The model under review builds one solid part; all positions refer to its coordinate system, in mm. Face numbers are marked on the shaded views. A direction names the side the tool comes from. Round coordinates to 2 decimals unless told otherwise and drop trailing zeros. Order: outer loops, then holes, each group sorted by start corner. A loop starts at its lowest first (then second) coordinate and runs counter-clockwise, first axis right, second up. Notation, with made-up numbers: M -16.75,-34 L -5.75,-34 A13 ccw -5.75,-19 Z; hole C 64,54 d11. An arc over 180 degrees is marked long. Answer as a JSON object with one key per item and string values. Group by question number.
1) For the marked faces 4, 5, 6 and 7, list the 3-axis set-ups (+Z, -Z, +X, -X, +Y, -Y) from which the entire face can be reached by the end or side of a thin tool; tool diameter is ignored.
2) The part is to be moulded in two halves that separate along X. For the marked faces 1, 2 and 3, say which applies: +X half, -X half, draft (parallel to the pull), parting line (faces both ways), or undercut.
3) Insertion check: pin 1 Ø0.5 at (y, z) = (6.5, 0) entering from -X (3 decimals); pin 2 Ø1.4 at (x, y) = (0, 6.5) entering from -Z; pin 3 Ø0.9 at (y, z) = (4, 0) entering from +X. Each pin has a flat end and moves straight along its axis. Give the tip position at first contact, or say it passes through.
4) Consider section A-A, the plane z = 0. Write out the cut boundary in (x, y) (1 decimal).
5) To check wall thickness, follow line 1 (Y direction, x = 0, z = 0) (3 decimals); line 2 (X direction, y = 4.25, z = -0.75); line 3 (Y direction, x = 0, z = -1.2). State the ranges of each line that lie inside material, in increasing order.
6) Consider section B-B, the plane x = 0. Write out the cut boundary in (y, z) (1 decimal), then the cut area to 3 significant figures.
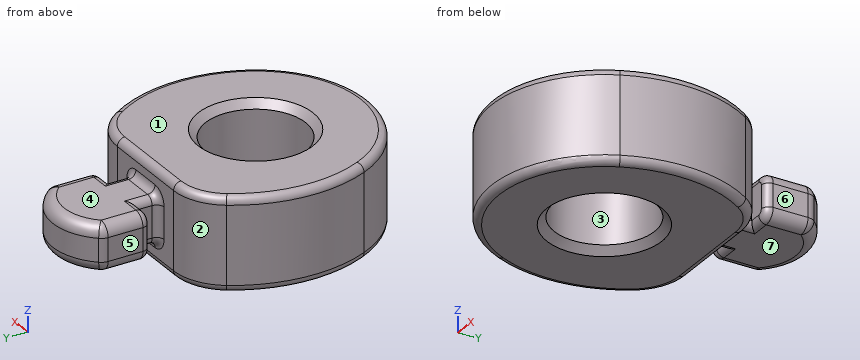
```python
from build123d import *

# Parameters (mm, degrees)
F1_DEPTH = 1.5875
F2_DEPTH = 3.175
F3_R     = 3.17499
F4_R     = 0.79375
F6_DEPTH = 3.175
F7_R     = 0.508
F8_R     = 0.508
F9_SIZE  = 0.508


# Not quite as in the source:
# - a fillet or chamfer is up to 0.001 mm smaller than in the source, because OpenCascade refuses the exact size
# - a feature names something its author has since deleted; it is built from what else it names


with BuildPart() as f1:
    # F0 (on Top) → F1 (new body, symmetric)
    with BuildSketch(Plane.XY):
        with BuildLine():
            Line((3.175, 4.7625), (3.175, 7.9375))
            ThreePointArc((3.175, 7.9375), (0, 9.525), (-3.175, 7.9375))
            Line((-3.175, 7.9375), (-3.175, 4.7625))
            Line((-3.175, 4.7625), (-1.5875, 4.7625))
            Line((-1.5875, 4.7625), (-1.5875, 3.175))
            Line((-1.5875, 3.175), (1.5875, 3.175))
            Line((1.5875, 3.175), (1.5875, 4.7625))
            Line((1.5875, 4.7625), (3.175, 4.7625))
        make_face()
    extrude(amount=F1_DEPTH, both=True)

    # F0 (on Top) → F2 (join, symmetric)
    with BuildSketch(Plane.XY):
        Polygon((6.35, 3.175), (1.5875, 3.175), (-1.5875, 3.175), (-6.35, 3.175), (-6.35, 0), (6.35, 0), align=None)
    extrude(amount=F2_DEPTH, both=True)

    # F3 (radius 3.175 in the source; OpenCascade refuses exactly that, so slightly less here)
    f3_edges = [f1.edges().sort_by_distance(p)[0] for p in [
        (6.35, 3.175, 0),
        (-6.35, 3.175, 0),
    ]]
    fillet(f3_edges, radius=F3_R)

    # F4
    f4_edges = [f1.edges().sort_by_distance(p)[0] for p in [
        (0, 9.525, -1.5875),
        (0, 9.525, 1.5875),
        (3.175, 6.35, -1.5875),
        (3.175, 6.35, 1.5875),
        (-3.175, 6.35, -1.5875),
        (-3.175, 6.35, 1.5875),
        (3.175, 7.9375, 0),
        (-3.175, 7.9375, 0),
    ]]
    fillet(f4_edges, radius=F4_R)

    # F5 (on Top) → F6 (join, symmetric)
    with BuildSketch(Plane.XY):
        with BuildLine():
            Line((1.5875, 3.175), (-1.5875, 3.175))
            ThreePointArc((-1.5875, 3.175), (-6.8727430801, -0.8804299989), (-7.0214355114, -7.540625))
            ThreePointArc((-7.0214355114, -7.540625), (0, -12.0715436111), (7.0214355114, -7.540625))
            ThreePointArc((7.0214355114, -7.540625), (6.8727430801, -0.8804299989), (1.5875, 3.175))
        make_face()
        with BuildLine():
            ThreePointArc((0, -0.936625), (3.429, -4.365625), (0, -7.794625))
            ThreePointArc((0, -7.794625), (-3.429, -4.365625), (0, -0.936625))
        make_face(mode=Mode.SUBTRACT)
        with BuildLine():
            Line((3.175, 3.175), (1.5875, 3.175))
            ThreePointArc((1.5875, 3.175), (6.8727430801, -0.8804299989), (7.0214355114, -7.540625))
            ThreePointArc((7.0214355114, -7.540625), (7.829384353, -2.9521060097), (6.3352448193, 1.4609241182))
            ThreePointArc((6.3352448193, 1.4609241182), (4.9725819485, 2.7188926062), (3.175, 3.175))
        make_face()
        with BuildLine():
            Line((-1.5875, 3.175), (-3.175, 3.175))
            ThreePointArc((-3.175, 3.175), (-4.9725819485, 2.7188926062), (-6.3352448193, 1.4609241182))
            ThreePointArc((-6.3352448193, 1.4609241182), (-7.829384353, -2.9521060097), (-7.0214355114, -7.540625))
            ThreePointArc((-7.0214355114, -7.540625), (-6.8727430801, -0.8804299989), (-1.5875, 3.175))
        make_face()
    extrude(amount=F6_DEPTH, both=True)

    # F7
    f7_edges = [f1.edges().sort_by_distance(p)[0] for p in [
        (0, 3.175, -1.5875),
        (-1.5875, 3.175, 0),
        (0, 3.175, 1.5875),
        (1.5875, 3.175, 0),
        (1.5875, 3.96875, 1.5875),
        (1.5875, 3.96875, -1.5875),
        (-1.5875, 3.96875, -1.5875),
        (-1.5875, 3.96875, 1.5875),
        (2.942516, 4.7625, 1.355016),
        (-2.942516, 4.7625, -1.355016),
    ]]
    fillet(f7_edges, radius=F7_R)

    # F8
    f8_edges = [f1.edges().sort_by_distance(p)[0] for p in [
        (-7.829384, -2.952106, -3.175),
        (-7.829384, -2.952106, 3.175),
        (0, 3.175, -3.175),
        (0, 3.175, 3.175),
        (-4.972586, 2.71889, -3.175),
        (0, -12.071544, -3.175),
        (7.829384, -2.952106, -3.175),
        (4.972586, 2.71889, -3.175),
        (4.972586, 2.71889, 3.175),
        (-4.972586, 2.71889, 3.175),
        (0, -12.071544, 3.175),
        (7.829384, -2.952106, 3.175),
    ]]
    fillet(f8_edges, radius=F8_R)

    # F9
    f9_edges = [f1.edges().sort_by_distance(p)[0] for p in [
        (0, -0.936625, 3.175),
        (0, -0.936625, -3.175),
    ]]
    chamfer(f9_edges, length=F9_SIZE)


solid = f1.part
```
Results list:
{
 "1": {"face 4": "+Z, +X, -X, +Y", "face 5": "+Z, -Z, -X, +Y", "face 6": "+Z, -Z, +X, +Y", "face 7": "-Z, +X, -X, +Y"},
 "2": {"face 1": "draft", "face 2": "-X half", "face 3": "undercut"},
 "3": {"pin 1": "x = -3.175", "pin 2": "z = -1.59", "pin 3": "x = 1.61"},
 "4": {"outline": "M -7,-7.5 A7.7 ccw 7,-7.5 A9.4 ccw 6.3,1.5 A3.8 ccw 3.2,3.2 L 2.1,3.2 A0.5 cw 1.6,3.7 L 1.6,4.8 L 2.7,4.8 A0.5 ccw 3.2,5.3 L 3.2,7.7 A0.8 ccw 3,8.2 A4 ccw -3,8.2 A0.8 ccw -3.2,7.7 L -3.2,5.3 A0.5 ccw -2.7,4.8 L -1.6,4.8 L -1.6,3.7 A0.5 cw -2.1,3.2 L -3.2,3.2 A3.8 ccw -6.3,1.5 A9.4 ccw Z; hole C 0,-4.4 d6.9"},
 "5": {"line 1": "-12.072 to -7.795, -0.937 to 9.525", "line 2": "-1.59 to 1.59", "line 3": "-12.07 to -7.79, -0.94 to 9.41"},
 "6": {"outline": "M -12.1,-2.7 A0.5 ccw -11.6,-3.2 L -8.3,-3.2 L -7.8,-2.7 L -7.8,2.7 L -8.3,3.2 L -11.6,3.2 A0.5 ccw -12.1,2.7 Z; M -0.9,-2.7 L -0.4,-3.2 L 2.7,-3.2 A0.5 ccw 3.2,-2.7 L 3.2,-2.1 A0.5 cw 3.7,-1.6 L 8.7,-1.6 A0.8 ccw 9.5,-0.8 L 9.5,0.8 A0.8 ccw 8.7,1.6 L 3.7,1.6 A0.5 cw 3.2,2.1 L 3.2,2.7 A0.5 ccw 2.7,3.2 L -0.4,3.2 L -0.9,2.7 Z", "area": "72.5 mm^2"}
}
